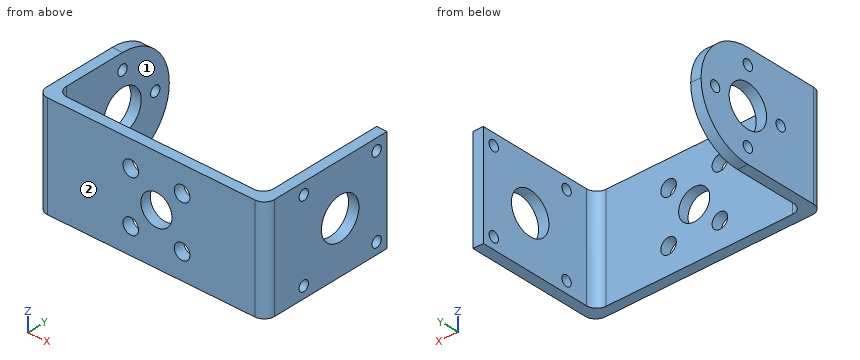
from build123d import *

# Parameters (mm, degrees)
EXTRUDE_1051_DEPTH     = 20
SKETCH2_R              = 4
SKETCH2_R_2            = 1
CUT_EXTRUDE_1_DEPTH    = 2
CUT_EXTRUDE_START      = -20
SKETCH3_R              = 1
SKETCH3_R_2            = 4
CUT_EXTRUDE_2_DEPTH    = 20
SKETCH4_R              = 3
SKETCH4_R_2            = 1.5
CUT_EXTRUDE_2789_DEPTH = 2
FILLET1_R              = 10
FILLET2_R              = 2


with BuildPart() as part:
    # Sketch1 → Extrude 1051 (new body)
    with BuildSketch(Plane.XY):
        Polygon((0, 0), (44, 0), (44, 26), (42, 26), (42, 2), (2, 2), (2, 26), (0, 26), align=None)
    extrude(amount=EXTRUDE_1051_DEPTH)

    # Sketch2 → Отверстия под ось и винты 1 (cut)
    with BuildSketch(Plane.ZY):
        with Locations((10, 16)):
            Circle(SKETCH2_R)
        with Locations((10, 23)):
            Circle(SKETCH2_R_2)
        with Locations((17, 16)):
            Circle(SKETCH2_R_2)
        with Locations((10, 9)):
            Circle(SKETCH2_R_2)
        with Locations((3, 16)):
            Circle(SKETCH2_R_2)
    extrude(amount=-CUT_EXTRUDE_1_DEPTH, mode=Mode.SUBTRACT)

    # Sketch3 → Отверстия под ось и винты 2 (cut)
    with BuildSketch(Plane(origin=(44, 0, 0), x_dir=(0, 0, -1), z_dir=(1, 0, 0)).offset(CUT_EXTRUDE_START)):
        with Locations((-17.778174593, 23.778174593)):
            Circle(SKETCH3_R)
        with Locations(Location((-10, 16, 0), (0, 0, 180))):
            Circle(SKETCH3_R_2)
        with Locations((-2.221825407, 23.778174593)):
            Circle(SKETCH3_R)
        with Locations((-2.221825407, 8.221825407)):
            Circle(SKETCH3_R)
        with Locations((-17.778174593, 8.221825407)):
            Circle(SKETCH3_R)
    extrude(amount=CUT_EXTRUDE_2_DEPTH, mode=Mode.SUBTRACT)

    # Sketch4 → Cut-Extrude 2789 (cut)
    with BuildSketch(Plane.XZ):
        with Locations(Location((23, 10, 0), (0, 0, 270))):
            Circle(SKETCH4_R)
        with Locations(Location((18.050252532, 5.050252532, 0), (0, 0, 270))):
            Circle(SKETCH4_R_2)
        with Locations(Location((27.949747468, 5.050252532, 0), (0, 0, 270))):
            Circle(SKETCH4_R_2)
        with Locations(Location((18.050252532, 14.949747468, 0), (0, 0, 270))):
            Circle(SKETCH4_R_2)
        with Locations(Location((27.949747468, 14.949747468, 0), (0, 0, 270))):
            Circle(SKETCH4_R_2)
    extrude(amount=-CUT_EXTRUDE_2789_DEPTH, mode=Mode.SUBTRACT)

    # Fillet1
    fillet1_edges = [part.edges().sort_by_distance(p)[0] for p in [
        (1, 26, 0),
        (1, 26, 20),
    ]]
    fillet(fillet1_edges, radius=FILLET1_R - 0.0001)  # a hair under: the kernel refuses the full size

    # Fillet2
    fillet2_edges = [part.edges().sort_by_distance(p)[0] for p in [
        (44, 0, 10),
        (0, 0, 10),
        (2, 2, 10),
        (42, 2, 10),
    ]]
    fillet(fillet2_edges, radius=FILLET2_R)


solid = part.part
Verification items for the finished model (mm, model axes). Face numbers are marked on the shaded views. A direction names the side the tool comes from. Coordinates: 2 decimals unless noted, no trailing zeros. Order: outer loops, then holes, each group sorted by start corner. A loop starts at its lowest first (then second) coordinate and runs counter-clockwise, first axis right, second up. Notation, with made-up numbers: M 24.5,83.25 L 64.5,83.25 A13 ccw 64.5,88.25 Z; hole C 41.25,44 d2. An arc over 180 degrees is marked long. Return JSON: item names as keys, results as strings.
1) Thickness scan on L1, parallel to X at y = 24, z = 11.5; L2, parallel to Y at x = 13.5, z = 12; L3, parallel to Y at x = 43.3, z = 10. Record the ranges inside material, lowest first. Write a range as [from, to].
Answer list:
{"L1": "[0, 2], [42, 44]", "L2": "[0, 2]", "L3": "[0.48, 12], [20, 26]"}
2) Access from +Z, -Z, +X, -X, +Y, -Y to the whole of each face (thin tool, end or side, straight path). Record for the marked faces 1 and 2.
Answer list:
{"face 1": "+Z, -Z, +Y", "face 2": "+Z, -Z, +X, -X, -Y"}
3) Cross-section at D-D, the plane z = 2.5. Record the boundary of the cut face in (x, y), and give its area (3 significant figures).
Answer list:
{"outline": "M 0,2 A2 ccw 2,0 L 42,0 A2 ccw 44,2 L 44,7.26 L 42,7.26 L 42,4 A2 cw 40,2 L 4,2 A2 cw 2,4 L 2,15.13 L 0,15.13 Z; M 0,16.87 L 2,16.87 L 2,22.61 L 0,22.61 Z; M 42,9.18 L 44,9.18 L 44,22.82 L 42,22.82 Z; M 42,24.74 L 44,24.74 L 44,26 L 42,26 Z", "area": "166 mm2"}
4) Cross-section at C-C, the plane z = 4.5. Record the boundary of the cut face in (x, y).
Answer list:
{"outline": "M 0,2 A2 ccw 2,0 L 16.65,0 L 16.65,2 L 4,2 A2 cw 2,4 L 2,24.35 L 0,24.35 Z; M 19.45,0 L 26.55,0 L 26.55,2 L 19.45,2 Z; M 29.35,0 L 42,0 A2 ccw 44,2 L 44,26 L 42,26 L 42,4 A2 cw 40,2 L 29.35,2 Z"}
5) Gauge pin test, flat ends, axial feed: pin 1 (8 mm diameter, centred on x = 28.5, z = 10, fed in from +Y); pin 2 (7 mm diameter, centred on y = 16, z = 10, fed in from +X); pin 3 (1.8 mm diameter, centred on y = 9, z = 10, fed in from -X). Record the tip position at first contact, or that the pin passes through.
Answer list:
{"pin 1": "y = 2", "pin 2": "through", "pin 3": "x = 42"}
6) Cross-section at A-A, the plane y = 11.25. Record the boundary of the cut face in (x, z), and give its area (3 significant figures).
Answer list:
{"outline": "M 0,0 L 2,0 L 2,20 L 0,20 Z; M 42,0 L 44,0 L 44,20 L 42,20 Z", "area": "80.0 mm2"}
7) Cross-section at B-B, the plane x = 23. Record the boundary of the cut face in (y, z), and give its area (3 significant figures).
Answer list:
{"outline": "M 0,0 L 2,0 L 2,7 L 0,7 Z; M 0,13 L 2,13 L 2,20 L 0,20 Z", "area": "28.0 mm2"}
